Input: part model. Units: mm. Frame: model coordinates. Coordinates: 2 decimals unless noted, no trailing zeros. Order: outer loops, then holes, each group sorted by start corner. A loop starts at its lowest first (then second) coordinate and runs counter-clockwise, first axis right, second up.
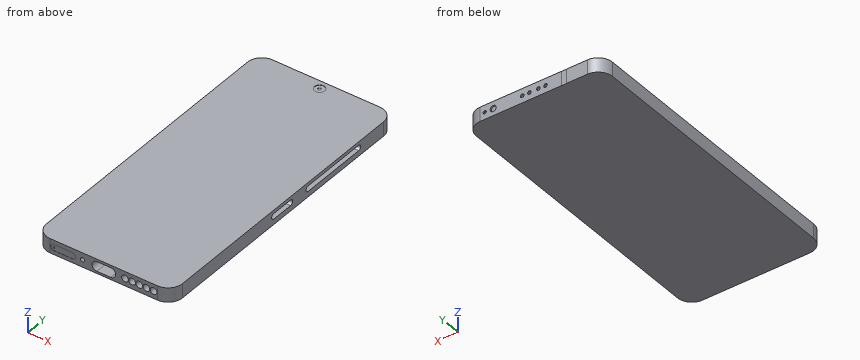
from build123d import *

# Parameters (mm, degrees)
EXTRUDE_2_DEPTH      = 10
SKETCH_10_R          = 1.25
SKETCH_10_R_2        = 2.1
SKETCH_10_R_3        = 1.15
CUT_EXTRUDE_3_DEPTH  = 1
CUT_EXTRUDE_4_DEPTH  = 20.085810478
SKETCH_16_R          = 1.45
SKETCH_16_R_2        = 2.328282895
CUT_EXTRUDE_6_DEPTH  = 10
SKETCH_18_R          = 0.54507581
CUT_EXTRUDE_7_DEPTH  = 10
CUT_EXTRUDE_8_DEPTH  = 8
SKETCH_22_R          = 3.550641332
CUT_EXTRUDE_9_DEPTH  = 0.2
SKETCH_23_R          = 1.070824202
CUT_EXTRUDE_10_DEPTH = 0.2
CUT_EXTRUDE_11_DEPTH = 0.1
SKETCH_8_W           = 3.574817698
SKETCH_8_H           = 10
CUT_EXTRUDE_13_DEPTH = 0.1


with BuildPart() as part:
    # 草图1 → 凸台-拉伸2 (new body)
    with BuildSketch(Plane.XY):
        with BuildLine():
            Line((-37.5, 105), (37.5, 105))
            ThreePointArc((37.5, 105), (44.571067812, 102.071067812), (47.5, 95))
            Line((47.5, 95), (47.5, -95))
            ThreePointArc((47.5, -95), (44.571067812, -102.071067812), (37.5, -105))
            Line((37.5, -105), (-37.5, -105))
            ThreePointArc((-37.5, -105), (-44.571067812, -102.071067812), (-47.5, -95))
            Line((-47.5, -95), (-47.5, 95))
            ThreePointArc((-47.5, 95), (-44.571067812, 102.071067812), (-37.5, 105))
        make_face()
    extrude(amount=EXTRUDE_2_DEPTH)

    # 草图10 → 切除-拉伸3 (cut)
    with BuildSketch(Plane(origin=(0, 105, 0), x_dir=(1, 0, 0), z_dir=(0, 1, 0))):
        with Locations(Location((-3.103218147, -5, 0), (0, 0, 270))):
            Circle(SKETCH_10_R)
        with Locations(Location((-8.103218147, -5, 0), (0, 0, 270))):
            Circle(SKETCH_10_R)
        with Locations(Location((8.103218147, -5, 0), (0, 0, 90))):
            Circle(SKETCH_10_R)
        with Locations(Location((3.103218147, -5, 0), (0, 0, 90))):
            Circle(SKETCH_10_R)
        with Locations(Location((28.429371283, -5, 0), (0, 0, 270))):
            Circle(SKETCH_10_R_2)
        with Locations(Location((34.368889588, -5, 0), (0, 0, 270))):
            Circle(SKETCH_10_R_3)
    extrude(amount=-CUT_EXTRUDE_3_DEPTH, mode=Mode.SUBTRACT)

    # 草图14 → 切除-拉伸4 (cut)
    with BuildSketch(Plane.XZ.offset(105)):
        with BuildLine():
            Line((-4.965024582, 8.276916224), (4.834975418, 8.276916224))
            ThreePointArc((4.834975418, 8.276916224), (8.211192134, 4.900699508), (4.834975418, 1.524482793))
            Line((4.834975418, 1.524482793), (-4.965024582, 1.524482793))
            ThreePointArc((-4.965024582, 1.524482793), (-8.341241297, 4.900699508), (-4.965024582, 8.276916224))
        make_face()
    extrude(amount=-CUT_EXTRUDE_4_DEPTH, mode=Mode.SUBTRACT)

    # 草图16 → 切除-拉伸6 (cut)
    with BuildSketch(Plane.XZ.offset(105)):
        with Locations(Location((-14.907323762, 5.165500819, 0), (0, 0, 270))):
            Circle(SKETCH_16_R)
        with Locations(Location((14.729603626, 5.165500819, 0), (0, 0, 270))):
            Circle(SKETCH_16_R_2)
        with Locations(Location((19.729603626, 5.165500819, 0), (0, 0, 270))):
            Circle(SKETCH_16_R_2)
        with Locations(Location((24.729603626, 5.165500819, 0), (0, 0, 270))):
            Circle(SKETCH_16_R_2)
        with Locations(Location((29.729603626, 5.165500819, 0), (0, 0, 270))):
            Circle(SKETCH_16_R_2)
        with Locations(Location((34.729603626, 5.165500819, 0), (0, 0, 270))):
            Circle(SKETCH_16_R_2)
    extrude(amount=-CUT_EXTRUDE_6_DEPTH, mode=Mode.SUBTRACT)

    # 草图18 → 切除-拉伸7 (cut)
    with BuildSketch(Plane.XZ.offset(105)):
        with Locations(Location((-34.978222052, 4.882313786, 0), (0, 0, 270))):
            Circle(SKETCH_18_R)
    extrude(amount=-CUT_EXTRUDE_7_DEPTH, mode=Mode.SUBTRACT)

    # 草图21 → 切除-拉伸8 (cut)
    with BuildSketch(Plane(origin=(47.5, 0, 0), x_dir=(0, 0, -1), z_dir=(1, 0, 0))):
        with BuildLine():
            Line((-3.80943092, 71.612022187), (-3.80943092, 23.612022187))
            ThreePointArc((-3.80943092, 23.612022187), (-5.70879523, 21.712657877), (-7.60815954, 23.612022187))
            Line((-7.60815954, 23.612022187), (-7.60815954, 71.612022187))
            ThreePointArc((-7.60815954, 71.612022187), (-5.70879523, 73.511386497), (-3.80943092, 71.612022187))
        make_face()
        with BuildLine():
            Line((-3.753848509, 7.202317814), (-3.753848509, -8.787308396))
            ThreePointArc((-3.753848509, -8.787308396), (-5.70879523, -10.742255117), (-7.663741952, -8.787308396))
            Line((-7.663741952, -8.787308396), (-7.663741952, 7.202317814))
            ThreePointArc((-7.663741952, 7.202317814), (-5.70879523, 9.157264535), (-3.753848509, 7.202317814))
        make_face()
    extrude(amount=-CUT_EXTRUDE_8_DEPTH, mode=Mode.SUBTRACT)

    # 草图22 → 切除-拉伸9 (cut)
    with BuildSketch(Plane.XY.offset(10)):
        with Locations((0, 98.825967342)):
            Circle(SKETCH_22_R)
    extrude(amount=-CUT_EXTRUDE_9_DEPTH, mode=Mode.SUBTRACT)

    # 草图23 → 切除-拉伸10 (cut)
    with BuildSketch(Plane.XY.offset(9.8)):
        with Locations((0, 98.825967342)):
            Circle(SKETCH_23_R)
    extrude(amount=-CUT_EXTRUDE_10_DEPTH, mode=Mode.SUBTRACT)

    # 草图19 → 切除-拉伸11 (cut)
    with BuildSketch(Plane.XZ.offset(105)):
        with BuildLine():
            Line((-34.978222052, 7.064787425), (-21.832097418, 7.064787425))
            ThreePointArc((-21.832097418, 7.064787425), (-19.64962378, 4.882313786), (-21.832097418, 2.699840148))
            Line((-21.832097418, 2.699840148), (-34.978222052, 2.699840148))
            ThreePointArc((-34.978222052, 2.699840148), (-37.160695691, 4.882313786), (-34.978222052, 7.064787425))
        make_face()
    extrude(amount=-CUT_EXTRUDE_11_DEPTH, mode=Mode.SUBTRACT)

    # 草图8 → 切除-拉伸13 (cut)
    with BuildSketch(Plane(origin=(0, 105, 0), x_dir=(1, 0, 0), z_dir=(0, 1, 0))):
        with Locations((-21, -5)):
            Rectangle(SKETCH_8_W, SKETCH_8_H)
    extrude(amount=-CUT_EXTRUDE_13_DEPTH, mode=Mode.SUBTRACT)


solid = part.part
Item 1: Ray query, probe 1 along Y at (x, z) = (0, 9.85); probe 2 along Y at (x, z) = (7.5, 5); probe 3 along Y at (x, z) = (-24, 6.5). Return the intervals inside material, ascending.
Response values:
probe 1: y = -105 to 95.28, 102.38 to 105
probe 2: y = -84.91 to 104
probe 3: y = -104.9 to 105
Item 2: Pin query (flat end, axial travel): pin 1 Ø10 at (x, y) = (-6, 81.5) entering from -Z; pin 2 Ø3 at (x, z) = (19.73, 5.17) entering from -Y; pin 3 Ø1.8 at (x, z) = (-21, 4) entering from +Y; pin 4 Ø2.5 at (x, y) = (0, 98.83) entering from +Z. Return the tip coordinate at first contact, or that it passes through.
Response values:
pin 1: stops at z = 0
pin 2: stops at y = -95
pin 3: stops at y = 104.9
pin 4: stops at z = 9.8
Item 3: Cut plane A-A on y = -87. Return loops of the section in (x, z), then the cut area to 3 significant figures.
Response values:
outline: (-47.5, 0) - (47.5, 0) - (47.5, 10) - (-47.5, 10) - close; hole (-4.97, 1.52) - (4.83, 1.52) arc R3.38 ccw to (4.83, 8.28) - (-4.97, 8.28) arc R3.38 ccw to start
area: 848 mm2
